```python
from build123d import *

# Parameters (mm, degrees)
SKETCH_1_R          = 40
SKETCH_1_R_2        = 33
EXTRUDE_1_DEPTH     = 4
EXTRUDE_START       = 8
SKETCH_2_R          = 40
SKETCH_2_R_2        = 36
EXTRUDE_2_DEPTH     = 8
EXTRUDE_3_DEPTH     = 3
SKETCH_5_R          = 1.05
SKETCH_5_R_2        = 1
SKETCH_5_R_3        = 2
CUT_EXTRUDE_1_DEPTH = 5
FILLET_1_R          = 10


with BuildPart() as part:
    # 草图1 → 凸台-拉伸1 (new body)
    with BuildSketch(Plane.XY):
        with Locations((-86.606649797, -63.783530386)):
            Circle(SKETCH_1_R)
        with Locations((-86.606649797, -63.783530386)):
            Circle(SKETCH_1_R_2, mode=Mode.SUBTRACT)
    extrude(amount=EXTRUDE_1_DEPTH)

    # 草图2 → 凸台-拉伸2 (add)
    with BuildSketch(Plane(origin=(0, 0, 0), x_dir=(-1, 0, 0), z_dir=(0, 0, -1)).offset(EXTRUDE_START)):
        with Locations((86.606649797, -63.783530386)):
            Circle(SKETCH_2_R)
        with Locations((86.606649797, -63.783530386)):
            Circle(SKETCH_2_R_2, mode=Mode.SUBTRACT)
    extrude(amount=-EXTRUDE_2_DEPTH)

    # 草图4 → 凸台-拉伸3 (add)
    with BuildSketch(Plane.XY.offset(4)):
        with BuildLine():
            Line((-103.161659788, 44.080644126), (-149.530913489, 25.375235519))
            Line((-149.530913489, 25.375235519), (-119.454633349, -49.181524695))
            ThreePointArc((-119.454633349, -49.181524695), (-100.016535475, -30.541466329), (-73.085379648, -30.476116088))
            Line((-73.085379648, -30.476116088), (-103.161659788, 44.080644126))
        make_face()
    extrude(amount=-EXTRUDE_3_DEPTH)

    # 草图5 → 切除-拉伸1 (cut)
    with BuildSketch(Plane(origin=(0, 0, 1), x_dir=(-1, 0, 0), z_dir=(0, 0, -1))):
        with Locations((113.059715781, -24.852893212)):
            Circle(SKETCH_5_R)
        with Locations((120.541879224, -6.305191731)):
            Circle(SKETCH_5_R)
        with Locations((101.994177743, 1.176971711)):
            Circle(SKETCH_5_R)
        with Locations((94.512014301, -17.370729769)):
            Circle(SKETCH_5_R)
        with Locations((116.800797503, -15.579042472)):
            Circle(SKETCH_5_R_2)
        with Locations((98.253096022, -8.096879029)):
            Circle(SKETCH_5_R_2)
        with Locations((103.785865041, -21.111811491)):
            Circle(SKETCH_5_R_2)
        with Locations((111.268028484, -2.56411001)):
            Circle(SKETCH_5_R_2)
        with Locations((114.369508098, 31.768673665)):
            Circle(SKETCH_5_R_3)
        with Locations((132.917209579, 24.286510222)):
            Circle(SKETCH_5_R_3)
        with Locations((119.902277117, 18.753741203)):
            Circle(SKETCH_5_R_3)
        with Locations((125.435046136, 5.738808742)):
            Circle(SKETCH_5_R_3)
        with Locations((106.887344656, 13.220972184)):
            Circle(SKETCH_5_R_3)
    extrude(amount=-CUT_EXTRUDE_1_DEPTH, mode=Mode.SUBTRACT)

    # 圆角1
    fillet_1_edges = [part.edges().sort_by_distance(p)[0] for p in [
        (-149.530913489, 25.375235519, 2.5),
        (-103.161659788, 44.080644126, 2.5),
    ]]
    fillet(fillet_1_edges, radius=FILLET_1_R)


solid = part.part
```
The model under review builds one solid part; all positions refer to its coordinate system, in mm. A direction names the side the tool comes from. Round coordinates to 2 decimals unless told otherwise and drop trailing zeros. Order: outer loops, then holes, each group sorted by start corner. A loop starts at its lowest first (then second) coordinate and runs counter-clockwise, first axis right, second up. Notation, with made-up numbers: (47, 23) -> (56, 23) arc R33 ccw to (56, 52) -> close; hole circle Ø5 at (69.25, 48.5). An arc over 180 degrees is marked (long way). Use a Markdown table: item, result.
Q1. We need section C-C on y = -87. Write out the cut boundary in (x, z).
Values:
| item | result |
|---|---|
| outline | (-119.18, -8) -> (-114.12, -8) -> (-114.12, 0) -> (-110.06, 0) -> (-110.06, 4) -> (-119.18, 4) -> close; (-63.15, 0) -> (-59.09, 0) -> (-59.09, -8) -> (-54.03, -8) -> (-54.03, 4) -> (-63.15, 4) -> close |
Q2. We need section B-B on x = -125. Write out the cut boundary in (y, z) (3 decimals), then the cut area to 3 significant figures.
Values:
| item | result |
|---|---|
| outline | (-75.006, -8) -> (-52.561, -8) -> (-52.561, 4) -> (-75.006, 4) -> close; (-35.435, 1) -> (3.787, 1) -> (3.787, 4) -> (-35.435, 4) -> close; (7.691, 1) -> (35.271, 1) -> (35.271, 4) -> (7.691, 4) -> close |
| area | 470 mm^2 |
Q3. Tool access review of faces 1 (the cylindrical face through (-127.343, 6.34, 2.479)), 2 (the flat face through (-57, -80, 0)), 3 (the flat face through (-133.8, -13.62, 2.52)): name each direction out of +Z, -Z, +X, -X, +Y, -Y from which nothing blocks a thin tool from reaching the whole face with its end or side.
Values:
| item | result |
|---|---|
| face 1 | +Z, -Z |
| face 2 | -Z |
| face 3 | +Z, -Z, -X |
Q4. We need section D-D on x = -106.5. Write out the cut boundary in (y, z), then the cut area to 3 significant figures.
Values:
| item | result |
|---|---|
| outline | (-98.49, -8) -> (-93.79, -8) -> (-93.79, 0) -> (-90.11, 0) -> (-90.11, 4) -> (-98.49, 4) -> close; (-37.45, 0) -> (-33.78, 0) -> (-33.78, -8) -> (-29.08, -8) -> (-29.08, 1) -> (11.26, 1) -> (11.26, 4) -> (-37.45, 4) -> close; (15.18, 1) -> (40.82, 1) -> (40.82, 4) -> (15.18, 4) -> close |
| area | 340 mm^2 |
Q5. Clearance check with flat-ended pins moving along their axes: P1, Ø1.9, axis at x = -101.99, y = 1.18, coming from the +Z side (3 decimals); P2, Ø5, axis at x = -62.5, z = -4.5, coming from the -Y side; P3, Ø5, axis at x = -125.44, y = 5.74, coming from the -Z side; P4, Ø1, axis at x = -133, z = 2, coming from the +Y side. State where each tip first meets the part, or that it passes through.
Values:
| item | result |
|---|---|
| P1 | passes through |
| P2 | stops at y = -97.45 |
| P3 | stops at z = 1 |
| P4 | stops at y = 32.25 |
Q6. Mouldability with a two-part tool opening along X and no side actions: class faces 4 (the cylindrical face through (-145.675, 23.856, 2.479)), 5 (the cylindrical face through (-116.277, 32.369, 2.479)), 6 (the cylindrical face through (-104.88, 40.31, 2.48)), 7 (the flat face through (-50.9, -57.7, -8)) as +X half, -X half, draft (parallel to the pull), parting line (faces both ways), or undercut.
Values:
| item | result |
|---|---|
| face 4 | -X half |
| face 5 | undercut |
| face 6 | parting line |
| face 7 | draft |
Q7. For line 1 (Y direction, x = -117, z = 2.5); line 2 (X direction, y = -43.5, z = 0.25); line 3 (Y direction, x = -101.5, z = 3), list the stretches that pass through material, from the lowest coordinate up.
Values:
| item | result |
|---|---|
| line 1 | y = -89.79 to -76.64, -50.93 to -16.56, -14.6 to 38.5 |
| line 2 | x = -121.08 to -112.64, -60.58 to -52.13 |
| line 3 | y = -100.91 to -93.23, -34.34 to 0.25, 2.1 to 38.01 |
Q8. We need section A-A on y = -32.5. Write out the cut boundary in (x, z).
Values:
| item | result |
|---|---|
| outline | (-126.18, 1) -> (-111.53, 1) -> (-111.53, -8) -> (-104.42, -8) -> (-104.42, 0) -> (-97.11, 0) -> (-97.11, 4) -> (-126.18, 4) -> close; (-76.1, 0) -> (-68.79, 0) -> (-68.79, -8) -> (-61.68, -8) -> (-61.68, 4) -> (-76.1, 4) -> close |
